```python
from build123d import *

# Parameters (mm, degrees)
SKETCH1_R                      = 88.9
BOSS_EXTRUDE1_DEPTH            = 3.175
SKETCH2_R                      = 12.065
BOSS_EXTRUDE2_DEPTH            = 3.175
SKETCH5_R                      = 10.4
CUT_EXTRUDE1_DEPTH             = 5.525
SKETCH6_R                      = 5
CUT_EXTRUDE2_DEPTH             = 4
CBORE_FOR_M2_SHCS1_D           = 2.2
CBORE_FOR_M2_SHCS1_DEPTH       = 6
CBORE_FOR_M2_SHCS1_CBORE_D     = 4.4
CBORE_FOR_M2_SHCS1_CBORE_DEPTH = 2
CBORE_FOR_M2_SHCS1_TIP         = 0.660946681
M4_CLEARANCE_HOLE1_D           = 4.5


with BuildPart() as part:
    # Sketch1 → Boss-Extrude1 (new, symmetric)
    with BuildSketch(Plane(origin=(0, 0, 0), x_dir=(1, 0, 0), z_dir=(0, 1, 0))):
        with Locations(Location((0, 0, 0), (0, 0, 270))):
            Circle(SKETCH1_R)
    extrude(amount=BOSS_EXTRUDE1_DEPTH, both=True)

    # Sketch2 → Boss-Extrude2 (add)
    with BuildSketch(Plane.XZ.offset(3.175)):
        with Locations(Location((0, 0, 0), (0, 0, 90))):
            Circle(SKETCH2_R)
    extrude(amount=BOSS_EXTRUDE2_DEPTH)

    # Sketch5 → Cut-Extrude1 (cut)
    with BuildSketch(Plane(origin=(0, 3.175, 0), x_dir=(1, 0, 0), z_dir=(0, 1, 0))):
        with Locations(Location((0, 0, 0), (0, 0, 270))):
            Circle(SKETCH5_R)
    extrude(amount=-CUT_EXTRUDE1_DEPTH, mode=Mode.SUBTRACT)

    # Sketch6 → Cut-Extrude2 (cut)
    with BuildSketch(Plane(origin=(0, -2.35, 0), x_dir=(1, 0, 0), z_dir=(0, 1, 0))):
        with Locations(Location((0, 0, 0), (0, 0, 270))):
            Circle(SKETCH6_R)
    extrude(amount=-CUT_EXTRUDE2_DEPTH, mode=Mode.SUBTRACT)

    # CBORE for M2 SHCS1
    with Locations(Plane(origin=(0, -2.35, 0), x_dir=(1, 0, 0), z_dir=(0, 1, 0))):
        with Locations((-5.65685425, 5.65685425), (0, 8), (5.65685425, 5.65685425), (8, 0), (5.65685425, -5.65685425), (0, -8), (-5.65685425, -5.65685425), (-8, 0)):
            CounterBoreHole(CBORE_FOR_M2_SHCS1_D / 2, CBORE_FOR_M2_SHCS1_CBORE_D / 2, CBORE_FOR_M2_SHCS1_CBORE_DEPTH, depth=CBORE_FOR_M2_SHCS1_DEPTH)
            with Locations((0, 0, -(CBORE_FOR_M2_SHCS1_DEPTH + CBORE_FOR_M2_SHCS1_TIP / 2))):  # 118° drill point
                Cone(0, CBORE_FOR_M2_SHCS1_D / 2, CBORE_FOR_M2_SHCS1_TIP, mode=Mode.SUBTRACT)

    # M4 Clearance Hole1 (through all)
    with Locations(Plane(origin=(0, 3.175, 0), x_dir=(1, 0, 0), z_dir=(0, 1, 0))):
        with Locations((19.05, -27.564242343), (-19.05, -27.564242343)):
            Hole(M4_CLEARANCE_HOLE1_D / 2)


solid = part.part
```
Model file for the job. Use its own axes, mm. A direction names the side the tool comes from. Coordinates: 2 decimals unless noted, no trailing zeros. Write each loop counter-clockwise with the first axis right and the second up, starting at its lowest first coordinate (ties: lowest second). Pieces come first, ordered by that corner, then holes. Notation, with made-up numbers: (79.5, 80) - (130.5, 80) arc R18 ccw to (130.5, 89) - close; hole circle Ø7 at (68, 67.25). An arc over 180 degrees is marked (long way). One line per item, written item: value. Start each with the question number.
1. Flat gauge pins, fed straight in: pin 1 (3 mm diameter, centred on y = 2, z = -65, fed in from +X); pin 2 (2 mm diameter, centred on x = -5, z = 6, fed in from +Y); pin 3 (16.5 mm diameter, centred on x = 0.5, z = 3.5, fed in from +Y) (3 decimals); pin 4 (5 mm diameter, centred on x = -35.5, y = -2.5, fed in from -Z). Where does each tip first touch, or does it go through?
2. Probe line 1 (Y direction, x = -22, z = -45.5) (3 decimals); line 2 (Z direction, x = 17, y = 1.5); line 3 (X direction, y = -0.75, z = 8). List the from-to ranges inside material, lowest first. Write a range as from..to.
3. Slice it at C-C (z = -73). Write the cut outline in (x, y) (3 decimals), plus the area to 3 significant figures.
4. Slice it at A-A (x = 19.05). Write the cut outline in (y, z) (3 decimals).
5. Tool access for faces 1 (the flat face through (-1, -4.35, -9)), 2 (the cylindrical face through (-4.88, -4.32, -1.08)): list every direction of +Z, -Z, +X, -X, +Y, -Y with a clear straight run to the whole face (end or side of a thin tool).
6. Slice it at B-B (z = 18). Write the cut outline in (x, y) (3 decimals).
7. Mould opens along X. For faces 3 (the cylindrical face through (-3.62, -4.74, 11.51)), 4 (the flat face through (5.2, -6.35, -0.2)), 5 (the flat face through (6, -4.35, -7)) say: released by +X, released by -X, zero draft, split by the parting line, or undercut.
Answers below:
1. pin 1: stops at x = 62.22
1. pin 2: stops at y = -4.35
1. pin 3: stops at y = 3.175
1. pin 4: stops at z = -82.55
2. line 1: y = -3.175..3.175
2. line 2: z = -87.26..26.64, 28.49..87.26
2. line 3: x = -88.54..-6.65, 6.65..88.54
3. outline: (-50.737, -3.175) - (50.737, -3.175) - (50.737, 3.175) - (-50.737, 3.175) - close
3. area: 644 mm^2
4. outline: (-3.175, -86.835) - (3.175, -86.835) - (3.175, 25.314) - (-3.175, 25.314) - close; (-3.175, 29.814) - (3.175, 29.814) - (3.175, 86.835) - (-3.175, 86.835) - close
5. face 1: +Y
5. face 2: +Y, -Y
6. outline: (-87.059, -3.175) - (87.059, -3.175) - (87.059, 3.175) - (-87.059, 3.175) - close
7. face 3: split by the parting line
7. face 4: zero draft
7. face 5: undercut
